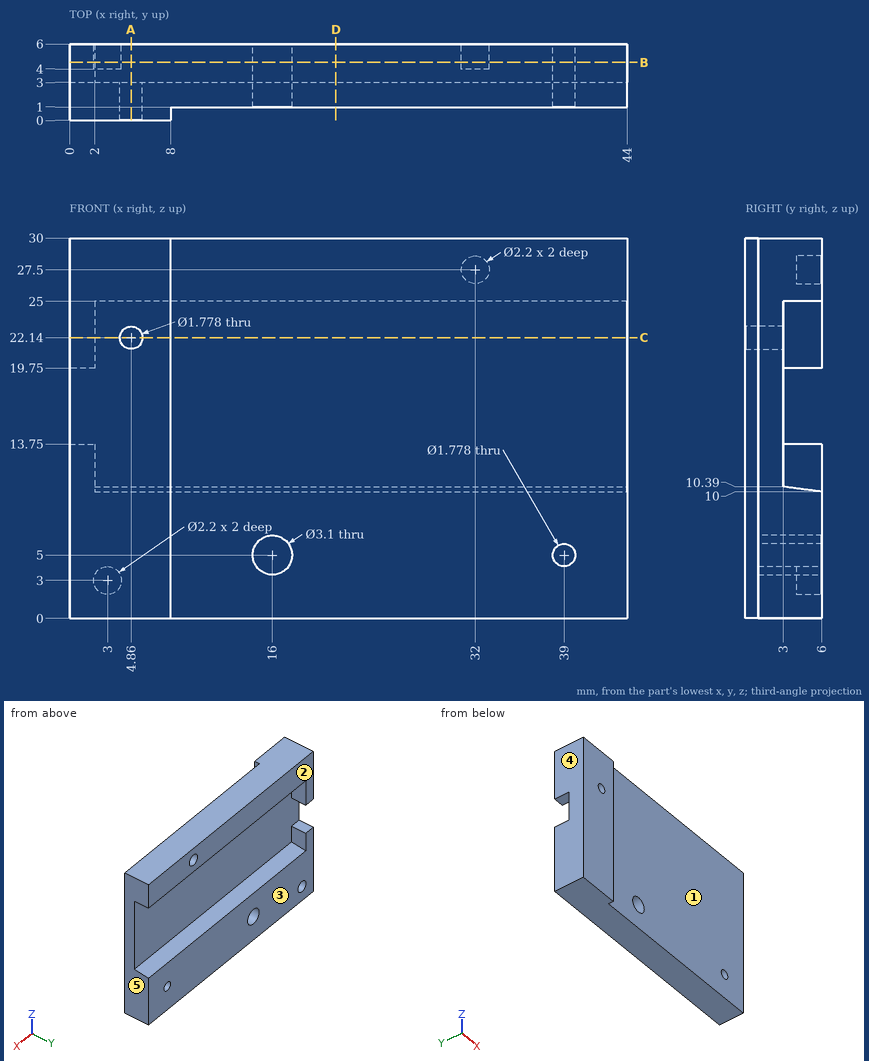
Answer from the drawing. Dimensions are ordinates in mm from the lowest x, y and z of the part. A direction names the side the tool comes from. Round coordinates to 2 decimals unless told otherwise and drop trailing zeros. Write each loop counter-clockwise with the first axis right and the second up, starting at its lowest first coordinate (ties: lowest second). Pieces come first, ordered by that corner, then holes. Notation, with made-up numbers: (54.25, -15.75) -> (102.25, -15.75) arc R12 cw to (102.25, -2.75) -> close; hole circle Ø9 at (14, 56.5). An arc over 180 degrees is marked (long way). Answer in a Markdown table with one row per item. Add a question column.
1) Determine the mould class of the marked faces 3, 4 and 5 for opening direction X: pulls with the +X half, pulls with the -X half, needs draft (parallel to the pull), parting line crosses it, or undercut.
2) Find section B-B, the plane y = 4.55. Determine the outline of the cut face in (x, z).
3) Given P1, Ø2.5, axis at y = 4.5, z = 12, coming from the +X side; P2, Ø1.1, axis at x = 3, z = 3, coming from the +Y side; P3, Ø11.5, axis at x = 13.5, z = 18.5, coming from the +Y side, each flat-ended and moving along its own axis, determine where each tip first touches the part or whether it passes through.
4) Find section A-A, the plane x = 4.86. Determine the outline of the cut face in (y, z), and give its area (3 significant figures).
5) Find section D-D, the plane x = 21. Determine the outline of the cut face in (y, z), and give its area (3 significant figures).
6) Which of the six approach directions +Z, -Z, +X, -X, +Y, -Y give full straight-line access (tool end or side, diameter ignored) to the marked faces 1 and 2?
7) Find section C-C, the plane z = 22.14. Determine the outline of the cut face in (x, y).
8) Consider line 1 (X direction, y = 2.5, z = 5); line 2 (X direction, y = 3.7, z = 5.5); line 3 (X direction, y = 2.25, z = 22.14). Determine where each line is inside the solid, lowest interval first.
Findings below:
| question | item | result |
|---|---|---|
| 1 | face 3 | needs draft |
| 1 | face 4 | pulls with the -X half |
| 1 | face 5 | pulls with the +X half |
| 2 | outline | (0, 0) -> (44, 0) -> (44, 10.19) -> (2, 10.19) -> (2, 13.75) -> (0, 13.75) -> close; (0, 19.75) -> (2, 19.75) -> (2, 25) -> (44, 25) -> (44, 30) -> (0, 30) -> close; hole circle Ø2.2 at (3, 3); hole circle Ø3.1 at (16, 5); hole circle Ø2.2 at (32, 27.5); hole circle Ø1.78 at (39, 5) |
| 3 | P1 | x = 2 |
| 3 | P2 | y = 4 |
| 3 | P3 | y = 3 |
| 4 | outline | (0, 0) -> (6, 0) -> (6, 10) -> (3, 10.39) -> (3, 21.25) -> (0, 21.25) -> close; (0, 23.03) -> (3, 23.03) -> (3, 25) -> (6, 25) -> (6, 30) -> (0, 30) -> close |
| 4 | area | 130 mm² |
| 5 | outline | (1, 0) -> (6, 0) -> (6, 10) -> (3, 10.39) -> (3, 25) -> (6, 25) -> (6, 30) -> (1, 30) -> close |
| 5 | area | 106 mm² |
| 6 | face 1 | +Z, -Z, +X, -Y |
| 6 | face 2 | +Z, -Z, +X, -X, +Y |
| 7 | outline | (0, 0) -> (3.97, 0) -> (3.97, 3) -> (2, 3) -> (2, 6) -> (0, 6) -> close; (5.75, 0) -> (8, 0) -> (8, 1) -> (44, 1) -> (44, 3) -> (5.75, 3) -> close |
| 8 | line 1 | 0 to 14.45, 17.55 to 38.11, 39.89 to 44 |
| 8 | line 2 | 0 to 14.53, 17.47 to 38.26, 39.74 to 44 |
| 8 | line 3 | 0 to 3.97, 5.75 to 44 |
